from build123d import *

# Parameters (mm, degrees)
CUT_EXTRUDE_1_DEPTH = 2
FILLET_1_R          = 0.2


with BuildPart() as part:
    # 草图1 → 旋转1 (revolve)
    with BuildSketch(Plane.XY):
        Polygon((0, 0), (0, 4.5), (3.5, 4.5), (3.5, 2.5), (11.5, 2.5), (11.5, 2), (19.5, 2), (19.5, 0), align=None)
    revolve(axis=Axis((19.5, 0, 0), (-1, 0, 0)))

    # 草图2 → 切除-拉伸1 (cut)
    with BuildSketch(Plane.ZY):
        Polygon((1.5, 0.866025404), (0, 1.732050808), (-1.5, 0.866025404), (-1.5, -0.866025404), (0, -1.732050808), (1.5, -0.866025404), align=None)
    extrude(amount=-CUT_EXTRUDE_1_DEPTH, mode=Mode.SUBTRACT)

    # 圆角1
    fillet_1_edges = [part.edges().sort_by_distance(p)[0] for p in [
        (3.5, -4.5, 0),
        (0, -4.5, 0),
    ]]
    fillet(fillet_1_edges, radius=FILLET_1_R)


solid = part.part
Check sheet for the modelled part. Datum: model origin and axes. Units: mm. A direction names the side the tool comes from. Give positions to 0.01 mm unless a question says otherwise; leave off trailing zeros. Write each loop counter-clockwise with the first axis right and the second up, starting at its lowest first coordinate (ties: lowest second). Pieces come first, ordered by that corner, then holes. Notation, with made-up numbers: (43.5, 49) -> (64.5, 49) arc R25 ccw to (64.5, 67) -> close; hole circle Ø5 at (6.25, 68.5). An arc over 180 degrees is marked (long way). Use one line per item in the form item = value. Start each with the question number.
1. Access from +Z, -Z, +X, -X, +Y, -Y to the whole of each face (thin tool, end or side, straight path). Record for faces 1 (the flat face through (19.5, 0, 0)), 2 (the flat face through (3.5, 2, 2)), 3 (the flat face through (1, 0, 1.5)).
2. Section check A-A (y = 0). Record the cut outline in (x, z), and give its area (3 significant figures).
3. Go/stop test with flat-tipped pins: P1, Ø3, axis at x = 10.5, z = 1.5, coming from the +Y side; P2, Ø3, axis at y = -3, z = -3.5, coming from the +X side; P3, Ø4, axis at x = 17.5, y = 3, coming from the -Z side. Record where each tip stops, or that it passes through.
4. Mould release check, pull along Y, two halves, no side actions. Record for faces 4 (the flat face through (0.986, -1.305, 0.74)), 5 (the cylindrical face through (1.77, -0.59, -4.46)), 6 (the flat face through (0, 0, 2)): pulls with the +Y half, pulls with the -Y half, needs draft (parallel to the pull), parting line crosses it, or undercut.
5. Section check C-C (x = 4.25). Record the cut outline in (y, z), and give its area (3 significant figures).
6. Section check B-B (x = 15.75). Record the cut outline in (y, z).
7. Thickness scan on line 1 along X through (y, z) = (3.5, -0.75); line 2 along X through (y, z) = (-1, 0.5); line 3 along Y through (x, z) = (17.75, 1). Record the ranges inside material, lowest first. Write a range as from..to.
Conclusion:
q1.face_1 = +Z, -Z, +X, +Y, -Y
q1.face_2 = +X
q1.face_3 = -X
q2.outline = (0, -4.3) arc R0.2 ccw to (0.2, -4.5) -> (3.3, -4.5) arc R0.2 ccw to (3.5, -4.3) -> (3.5, -2.5) -> (11.5, -2.5) -> (11.5, -2) -> (19.5, -2) -> (19.5, 2) -> (11.5, 2) -> (11.5, 2.5) -> (3.5, 2.5) -> (3.5, 4.3) arc R0.2 ccw to (3.3, 4.5) -> (0.2, 4.5) arc R0.2 ccw to (0, 4.3) -> (0, 1.5) -> (2, 1.5) -> (2, -1.5) -> (0, -1.5) -> close
q2.area = 97.5 mm²
q3.P1 = 2.5
q3.P2 = 3.5
q3.P3 = -1.73
q4.face_4 = undercut
q4.face_5 = parting line crosses it
q4.face_6 = needs draft
q5.outline = circle Ø5 at (0, 0)
q5.area = 19.6 mm²
q6.outline = circle Ø4 at (0, 0)
q7.line_1 = 0..3.5
q7.line_2 = 2..19.5
q7.line_3 = -1.73..1.73
